```python
from build123d import *

# Parameters (mm, degrees)
SKETCH1_R           = 7.5
BOSS_EXTRUDE1_DEPTH = 1.8
BOSS_EXTRUDE2_START = -18.8
SKETCH1_3_R         = 7.5
BOSS_EXTRUDE2_DEPTH = 18.8
BOSS_EXTRUDE3_DEPTH = 0.9
FILLET1_R           = 6
FILLET2_R           = 2


with BuildPart() as part:
    # Sketch1 → Boss-Extrude1 (new body)
    with BuildSketch(Plane(origin=(0, 0, 0), x_dir=(1, 0, 0), z_dir=(0, 1, 0))):
        with Locations(Location((0, 0, 0), (0, 0, 270))):
            Circle(SKETCH1_R)
    extrude(amount=BOSS_EXTRUDE1_DEPTH)

    # Sketch1_3 → Boss-Extrude2 (add)
    with BuildSketch(Plane(origin=(0, 0, 0), x_dir=(1, 0, 0), z_dir=(0, 1, 0)).offset(BOSS_EXTRUDE2_START)):
        with Locations(Location((0, 0, 0), (0, 0, 270))):
            Circle(SKETCH1_3_R)
    extrude(amount=BOSS_EXTRUDE2_DEPTH)

    # Sketch3 → Boss-Extrude3 (add)
    with BuildSketch(Plane(origin=(0, 1.8, 0), x_dir=(1, 0, 0), z_dir=(0, 1, 0))):
        Polygon((0, 50), (-10, -7.5), (10, -7.5), align=None)
    extrude(amount=-BOSS_EXTRUDE3_DEPTH)

    # Fillet1
    fillet1_edges = [part.edges().sort_by_distance(p)[0] for p in [
        (10, 1.35, 7.5),
    ]]
    fillet(fillet1_edges, radius=FILLET1_R)

    # Fillet2
    fillet2_edges = [part.edges().sort_by_distance(p)[0] for p in [
        (-10, 1.35, 7.5),
    ]]
    fillet(fillet2_edges, radius=FILLET2_R)


solid = part.part
```
The listing builds one solid part. Answer for the finished solid, in the listing's coordinates (mm). A direction names the side the tool comes from. Round coordinates to 2 decimals unless told otherwise and drop trailing zeros. Loops run counter-clockwise (first coordinate to the right, second up) from the corner with the lowest first, then second, coordinate; pieces in that order, holes last. Notation, with made-up numbers: (7.25, 4.25) - (34.25, 4.25) arc R24 ccw to (34.25, 40.25) - close; hole circle Ø5 at (12.5, -29). An arc over 180 degrees is marked (long way). Use one line per item in the form item = value. Start each with the question number.
1. The part is cut by section D-D on z = -31. Determine the outline of the cut face in (x, y), then the cut area to 3 significant figures.
2. Consider line 1 (Y direction, x = 2.25, z = -14); line 2 (Z direction, x = 0.25, y = -2.5); line 3 (Z direction, x = 3.75, y = -1.25). Determine where each line is inside the solid, lowest interval first. Write a range as [from, to].
3. A tool of negligible diameter and unlimited length cuts with its end or side. For faces 1 (the face through (0.33, -9.088, -7.493)), 2 (the face through (0, -18.8, 0)), from which of +Z, -Z, +X, -X, +Y, -Y can it reach the whole face along a straight path? Write none if from no direction.
4. The part is cut by section A-A on x = -1.25. Determine the outline of the cut face in (y, z), then the cut area to 3 significant figures.
5. Given pin 1 Ø3 at (x, z) = (-6, -14.5) entering from -Y; pin 2 Ø8 at (x, y) = (-6.5, -9) entering from +Z; pin 3 Ø3 at (x, y) = (0, -4) entering from -Z, each flat-ended and moving along its own axis, determine where each tip first touches the part or whether it passes through.
6. The part is cut by section B-B on z = -4.5. Determine the outline of the cut face in (x, y), then the cut area to 3 significant figures.
7. The part is cut by section C-C on y = -6. Determine the outline of the cut face in (x, z).
Geometry check:
q1.outline = (-3.3, 0.9) - (3.3, 0.9) - (3.3, 1.8) - (-3.3, 1.8) - close
q1.area = 5.95 mm^2
q2.line_1 = [0.9, 1.8]
q2.line_2 = [-7.5, 7.5]
q2.line_3 = [-6.5, 6.5]
q3.face_1 = -Y
q3.face_2 = +Z, -Z, +X, -X, -Y
q4.outline = (-18.8, -7.4) - (0.9, -7.4) - (0.9, -42.81) - (1.8, -42.81) - (1.8, 7.5) - (0.9, 7.5) - (0.9, 7.4) - (-18.8, 7.4) - close
q4.area = 337 mm^2
q5.pin_1 = 0.9
q5.pin_2 = 7.07
q5.pin_3 = -7.5
q6.outline = (-7.91, 0.9) - (-6, 0.9) - (-6, -18.8) - (6, -18.8) - (6, 0.9) - (7.91, 0.9) - (7.91, 1.8) - (-7.91, 1.8) - close
q6.area = 251 mm^2
q7.outline = circle Ø15 at (0, 0)
